The listing builds one solid part. Answer for the finished solid, in the listing's coordinates (mm). A direction names the side the tool comes from. Round coordinates to 2 decimals unless told otherwise and drop trailing zeros. Write each loop counter-clockwise with the first axis right and the second up, starting at its lowest first coordinate (ties: lowest second). Pieces come first, ordered by that corner, then holes. Notation, with made-up numbers: M -12.5,20.5 L -3.5,20.5 A9 ccw -3.5,32.5 Z; hole C 71,63 d2. An arc over 180 degrees is marked long. Put each result on its own line as item: value. Start each with the question number.
```python
from build123d import *

# Parameters (mm, degrees)
SKETCH001_W     = 188.75
SKETCH001_H     = 60.758838
SKETCH001_R     = 2.182812
PAD_DEPTH       = 3
PAD001_DEPTH    = 105.6
SKETCH004_W     = 328.820023
SKETCH004_H     = 275.658927
POCKET_DEPTH    = 200
SKETCH002_W     = 158.75
SKETCH002_H     = 72.39
PAD002_DEPTH    = 3
SKETCH003_R     = 1.4
PAD003_DEPTH    = 10
SKETCH005_R     = 7.5
POCKET001_DEPTH = 24.440644


with BuildPart() as part:
    # Sketch001 → Pad (new body)
    with BuildSketch(Plane.XY):
        with Locations((0, -5.939775)):
            Rectangle(SKETCH001_W, SKETCH001_H)
        with Locations((88.718146, 18.78279)):
            Circle(SKETCH001_R, mode=Mode.SUBTRACT)
        with Locations((88.718146, -30.66234)):
            Circle(SKETCH001_R, mode=Mode.SUBTRACT)
        with Locations((-88.718146, -30.66234)):
            Circle(SKETCH001_R, mode=Mode.SUBTRACT)
        with Locations((-88.718146, 18.78279)):
            Circle(SKETCH001_R, mode=Mode.SUBTRACT)
    extrude(amount=-PAD_DEPTH)

    # Sketch → Pad001 (join)
    with BuildSketch(Plane.XY):
        Polygon((73.375, -21.319194), (79.375, -21.319194), (79.375, 9.439644), (-79.375, 9.439644), (-79.375, -21.319194), (-73.375, -21.319194), (-73.375, 3.439644), (73.375, 3.439644), align=None)
    extrude(amount=PAD001_DEPTH)

    # Sketch004 (on DatumPlane) → Pocket (cut)
    with BuildSketch(Plane(origin=(0, -35, 0), x_dir=(1, 0, 0), z_dir=(0, -0.939693, 0.34202))):
        with Locations((-2.626228, 137.829464)):
            Rectangle(SKETCH004_W, SKETCH004_H)
    extrude(amount=POCKET_DEPTH, mode=Mode.SUBTRACT)

    # Sketch002 (on DatumPlane) → Pad002 (join)
    with BuildSketch(Plane(origin=(0, -35, 0), x_dir=(1, 0, 0), z_dir=(0, -0.939693, 0.34202))):
        with Locations((0, 76.195)):
            Rectangle(SKETCH002_W, SKETCH002_H)
    extrude(amount=-PAD002_DEPTH)

    # Sketch003 (on DatumPlane) → Pad003 (join)
    with BuildSketch(Plane(origin=(0, -35, 0), x_dir=(1, 0, 0), z_dir=(0, -0.939693, 0.34202))):
        with Locations((-75.565, 108.58)):
            Circle(SKETCH003_R)
        with Locations((75.565, 108.58)):
            Circle(SKETCH003_R)
        with Locations((75.565, 43.81)):
            Circle(SKETCH003_R)
        with Locations((-75.565, 43.81)):
            Circle(SKETCH003_R)
    extrude(amount=PAD003_DEPTH)

    # Sketch005 → Pocket001 (cut, through all)
    with BuildSketch(Plane.XZ):
        with Locations((0, 20)):
            Circle(SKETCH005_R)
    extrude(amount=-POCKET001_DEPTH, mode=Mode.SUBTRACT)


solid = part.part
```
Item 1: Consider line 1 along X through (y, z) = (-1.5, 46) (3 decimals); line 2 along Z through (x, y) = (0, 6); line 3 along Z through (x, y) = (-81, -15). Determine where each line is inside the solid, lowest interval first. Write a range as [from, to].
Item 2: Determine the mould class of faces 5 (the flat face through (-76, -21.319, 19)), 6 (the flat face through (-1, -6, 0)), 7 (the flat face through (73.375, -6, 37)), 8 (the flat face through (-79.375, -4, 38)) for opening direction X: released by +X, released by -X, zero draft, split by the parting line, or undercut.
Item 3: Section C-C (y = -12) is taken. Give the vertices of the cut face in (x, z) (3 decimals), and give its area (3 significant figures).
Item 4: Flat-ended cylindrical pins translate along their axes: pin 1 (6.5 mm diameter, centred on x = -77, z = 20.5, fed in from -Y); pin 2 (1 mm diameter, centred on y = -15, z = 21, fed in from +X) (3 decimals); pin 3 (3.5 mm diameter, centred on x = 88.72, y = -30.66, fed in from -Z); pin 4 (2 mm diameter, centred on y = -18.5, z = 43, fed in from -X) (3 decimals). Find the tip coordinate at first contact, or state that the pin passes through.
Item 5: Which of the six approach directions +Z, -Z, +X, -X, +Y, -Y give full straight-line access (tool end or side, diameter ignored) to faces 1 (the flat face through (-1, 3.44, 48)), 2 (the flat face through (76, -21.319, 19)), 3 (the flat face through (-1, -6, -3)), 4 (the flat face through (79.375, -4, 38))?
Item 6: Section D-D (z = 7.5) is taken. Give the vertices of the cut face in (x, y) (3 decimals), and give its area (3 significant figures).
Item 7: Section B-B (z = 20) is taken. Give the vertices of the cut face in (x, y) (3 decimals).
Output values:
1. line 1: x = [-79.375, -73.375], [73.375, 79.375]
1. line 2: z = [-3, 12.5], [27.5, 105.6]
1. line 3: z = [-3, 0]
2. face 5: zero draft
2. face 6: undercut
2. face 7: undercut
2. face 8: released by -X
3. outline: M -94.375,-3 L 94.375,-3 L 94.375,0 L 79.375,0 L 79.375,63.192 L -79.375,63.192 L -79.375,0 L -94.375,0 Z; hole M -73.375,0 L 73.375,0 L 73.375,54.421 L -73.375,54.421 Z
3. area: 2,610 mm^2
4. pin 1: stops at y = -21.32
4. pin 2: stops at x = 79.375
4. pin 3: passes through
4. pin 4: stops at x = -79.375
5. face 1: none
5. face 2: +X, -X, -Y
5. face 3: -Z, +X, -X, +Y, -Y
5. face 4: +Z, +X, +Y, -Y
6. outline: M -79.375,-21.319 L -73.375,-21.319 L -73.375,3.44 L 73.375,3.44 L 73.375,-21.319 L 79.375,-21.319 L 79.375,9.44 L -79.375,9.44 Z
6. area: 1,250 mm^2
7. outline: M -79.375,-21.319 L -73.375,-21.319 L -73.375,3.44 L -7.5,3.44 L -7.5,9.44 L -79.375,9.44 Z; M 7.5,3.44 L 73.375,3.44 L 73.375,-21.319 L 79.375,-21.319 L 79.375,9.44 L 7.5,9.44 Z
